Autodesk Inventor part; units mm, degrees
ref_plane "YZ Plane" through (0, 0, 0) normal (1, 0, 0) x (0, 1, 0)
ref_plane "XZ Plane" through (0, 0, 0) normal (0, 1, 0) x (-1, 0, 0)
ref_plane "XY Plane" through (0, 0, 0) normal (0, 0, 1) x (1, 0, 0)
sketch "Sketch1" plane through (0, 0, 0) normal (0, 0, 1) x (1, 0, 0)
  line L0 (0, 0) -> (0, 42.4688)
  line L1 (4.0132, 46.482) -> (45.6692, 46.482)
  line L2 (49.6824, 42.4688) -> (49.6824, 0)
  arc A0 (4.0132, 46.482) -> (0, 42.4688) centre (4.0132, 42.4688) ccw
  arc A1 (49.6824, 42.4688) -> (45.6692, 46.482) centre (45.6692, 42.4688) ccw
  line L3 (47.7012, 0) -> (47.7012, 42.4688)
  arc A2 (47.7012, 42.4688) -> (45.6692, 44.5008) centre (45.6692, 42.4688) ccw
  line L4 (45.6692, 44.5008) -> (4.0132, 44.5008)
  arc A3 (4.0132, 44.5008) -> (1.9812, 42.4688) centre (4.0132, 42.4688) ccw
  line L5 (1.9812, 42.4688) -> (1.9812, 0)
  line L6 (0, 0) -> (1.9812, 0)
  line L7 (47.7012, 0) -> (49.6824, 0)
  dimension "d1" = 1.9812
  dimension "d3" = 46.482
  dimension "d6" = 45.72
  dimension "d7" = 2.032
extrude "Extrusion1" add sketch "Sketch1" along normal blind 152.4
fillet "Fillet1" radius 3.175 4 edges at (0.9906, 0, 152.4) (48.6918, 0, 152.4) (48.6918, 0, 0) (0.9906, 0, 0)
hole "Hole1" at (49.6824, 23.241, 133.35) direction (-1, 0, 0) diameter 6.985 end through all
pattern_linear "Rectangular Pattern1" count 2 spacing 114.3 along (0, 0, -1) of "Hole1"
properties part number "GE-12052_modified"
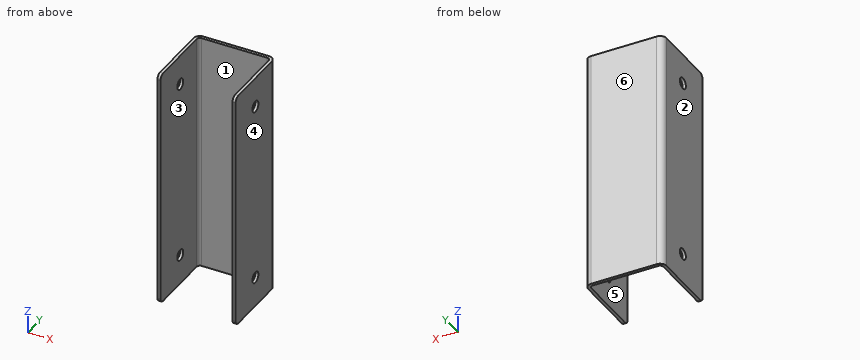
Input: part model. Units: mm. Frame: model coordinates. Face numbers are marked on the shaded views. A direction names the side the tool comes from. Round coordinates to 2 decimals unless told otherwise and drop trailing zeros. Order: outer loops, then holes, each group sorted by start corner. A loop starts at its lowest first (then second) coordinate and runs counter-clockwise, first axis right, second up.
1. Cut plane B-B, the plane z = 133.35. Output: boundary loops of the cut face in (x, y).
The answers:
outline: (0, 0) - (1.98, 0) - (1.98, 19.75) - (0, 19.75) - close; (0, 26.73) - (1.98, 26.73) - (1.98, 42.47) arc R2.03 cw to (4.01, 44.5) - (45.67, 44.5) arc R2.03 cw to (47.7, 42.47) - (47.7, 26.73) - (49.68, 26.73) - (49.68, 42.47) arc R4.01 ccw to (45.67, 46.48) - (4.01, 46.48) arc R4.01 ccw to (0, 42.47) - close; (47.7, 0) - (49.68, 0) - (49.68, 19.75) - (47.7, 19.75) - close
2. Pin query (flat end, axial travel): P1, Ø4, axis at x = 32.5, z = 87.5, coming from the -Y side. Return the tip coordinate at first contact, or that it passes through.
The answers:
P1: stops at y = 44.5
3. Cut plane C-C, the plane x = 23. Output: boundary loops of the cut face in (y, z).
The answers:
outline: (44.5, 0) - (46.48, 0) - (46.48, 152.4) - (44.5, 152.4) - close
4. Material intervals for line 1 (X direction, y = 8, z = 96); line 2 (Y direction, x = 34, z = 53); line 3 (Y direction, x = 48.7, z = 19.05), sorted ascending.
The answers:
line 1: x = 0 to 1.98, 47.7 to 49.68
line 2: y = 44.5 to 46.48
line 3: y = 0 to 19.75, 26.73 to 45.1
5. Cut plane A-A, the plane y = 18. Output: boundary loops of the cut face in (x, z), then the cut area to 3 significant figures.
The answers:
outline: (0, 0) - (1.98, 0) - (1.98, 152.4) - (0, 152.4) - close; (47.7, 0) - (49.68, 0) - (49.68, 152.4) - (47.7, 152.4) - close
area: 604 mm2
6. Mould query, pull axis X, two halves, no side actions, for the marked faces 1, 2, 3 and 4. Classes: released by +X, released by -X, zero draft, split by the parting line, or undercut.
The answers:
face 1: undercut
face 2: released by -X
face 3: undercut
face 4: released by +X
7. Set-up query: the marked faces 5 and 6. Return all of +Z, -Z, +X, -X, +Y, -Y with unobstructed straight access to the full face (end or side cutting, diameter ignored); none if empty.
The answers:
face 5: +Z, -Z, -Y
face 6: +Z, -Z, +X, -X, +Y
